Geometry: final body of the model. Coordinates: model frame, mm. A direction names the side the tool comes from. Give positions to 0.01 mm unless a question says otherwise; leave off trailing zeros. Order: outer loops, then holes, each group sorted by start corner. A loop starts at its lowest first (then second) coordinate and runs counter-clockwise, first axis right, second up. Notation, with made-up numbers: (-11, 5.25) -> (28, 5.25) arc R20 ccw to (28, 29.25) -> close; hole circle Ø2 at (-14.5, 77.5). An arc over 180 degrees is marked (long way). Answer in a Markdown table with one row per item. Add a question column.
Q1. Cut plane C-C on y = 2.25. Count the separate pieces of the cut face and the enclosed holes in it, and give its area (3 significant figures).
Q2. Set-up query: faces 4 (the face through (45, -4, 0)), 5 (the face through (-3.75, 2, -8)), 6 (the face through (19, 2.5, 10.5)). Return all of +Z, -Z, +X, -X, +Y, -Y with unobstructed straight access to the full face (end or side cutting, diameter ignored); none if empty.
Q3. Cut plane B-B on z = 0. Return the cut outline in (x, y), and give its area (3 significant figures).
Q4. Line query: line 1 along X through (y, z) = (1.6, 0); line 2 along X through (y, z) = (1.5, -8); line 3 along Z through (x, y) = (11.25, 1.25). Output: solid intervals per line, ascending. Write a range as from..to.
Q5. Contact query for flat-ended pins moving along their axis: P1, Ø1.5, axis at x = 10, y = 1.5, coming from the -Z side; P2, Ø2.5, axis at x = -10, y = 3.5, coming from the +Z side; P3, Ø1, axis at y = -2.5, z = -4, coming from the -X side; P4, Ø2, axis at x = 11.25, z = 0, coming from the -Y side. Output: stop coordinate, or through.
Q6. Cut plane D-D on x = 45.5. Return the cut outline in (y, z).
Q7. Pull-direction query (X, two-part tool) for faces 1 (the face through (11, 2, -9)), 2 (the face through (56.64, 2.54, 11.1)), 3 (the face through (-48.14, 2.54, 11.1)); classes: +X half, -X half, draft (parallel to the pull), parting line (faces both ways), or undercut.
Q8. Cut plane A-A on x = 11.25. Return the cut outline in (y, z).
from build123d import *

# Parameters (mm, degrees)
BOSS_EXTRUDE1_DEPTH = 5
SKETCH5_R           = 5
BOSS_EXTRUDE2_DEPTH = 4
SKETCH7_W           = 35
SKETCH7_H           = 3
CUT_EXTRUDE2_DEPTH  = 59.951251047
SKETCH6_W           = 7.5
SKETCH6_H           = 3
CUT_EXTRUDE1_DEPTH  = 59.951251047
SKETCH8_R           = 1.75
CUT_EXTRUDE3_DEPTH  = 59.951251047
FILLET3_R           = 3
FILLET2_R           = 0.25
CHAMFER1_SIZE       = 3


with BuildPart() as part:
    # Sketch1 → Boss-Extrude1 (new body)
    with BuildSketch(Plane(origin=(0, 0, 0), x_dir=(1, 0, 0), z_dir=(0, 1, 0))):
        Polygon((0, 12), (57.5, 12), (57.5, -12), (0, -12), (-49, -12), (-49, 12), align=None)
    extrude(amount=BOSS_EXTRUDE1_DEPTH)

    # Sketch5 → Boss-Extrude2 (add)
    with BuildSketch(Plane(origin=(0, 0, 0), x_dir=(1, 0, 0), z_dir=(0, 1, 0))):
        with Locations(Location((-37, 0, 0), (0, 0, 270))):
            Circle(SKETCH5_R)
        with Locations(Location((45.5, 0, 0), (0, 0, 90))):
            Circle(SKETCH5_R)
    extrude(amount=-BOSS_EXTRUDE2_DEPTH)

    # Sketch7 → Cut-Extrude2 (cut, through all)
    with BuildSketch(Plane.XZ):
        with Locations((0, 10.5)):
            Rectangle(SKETCH7_W, SKETCH7_H)
        with Locations((0, -10.5)):
            Rectangle(SKETCH7_W, SKETCH7_H)
    extrude(amount=-CUT_EXTRUDE2_DEPTH, mode=Mode.SUBTRACT)

    # Sketch6 → Cut-Extrude1 (cut, through all)
    with BuildSketch(Plane.XZ):
        with Locations((0, 7.5)):
            Rectangle(SKETCH6_W, SKETCH6_H)
        with Locations((0, -7.5)):
            Rectangle(SKETCH6_W, SKETCH6_H)
    extrude(amount=-CUT_EXTRUDE1_DEPTH, mode=Mode.SUBTRACT)

    # Sketch8 → Cut-Extrude3 (cut, through all)
    with BuildSketch(Plane.XZ):
        with Locations(Location((-11.25, 0, 0), (0, 0, 270))):
            Circle(SKETCH8_R)
        with Locations(Location((11.25, 0, 0), (0, 0, 90))):
            Circle(SKETCH8_R)
    extrude(amount=-CUT_EXTRUDE3_DEPTH, mode=Mode.SUBTRACT)

    # Fillet3
    fillet3_edges = [part.edges().sort_by_distance(p)[0] for p in [
        (-49, 2.5, 12),
        (-49, 2.5, -12),
        (57.5, 2.5, -12),
        (57.5, 2.5, 12),
    ]]
    fillet(fillet3_edges, radius=FILLET3_R)

    # Fillet2
    fillet2_edges = [part.edges().sort_by_distance(p)[0] for p in [
        (-37, -4, -5),
        (45.5, -4, 5),
    ]]
    fillet(fillet2_edges, radius=FILLET2_R)

    # Chamfer1
    chamfer1_edges = [part.edges().sort_by_distance(p)[0] for p in [
        (17.5, 2.5, 12),
        (-17.5, 2.5, 12),
        (17.5, 2.5, -12),
        (-17.5, 2.5, -12),
    ]]
    chamfer(chamfer1_edges, length=CHAMFER1_SIZE - 0.0001)  # a hair under: the kernel refuses the full size


solid = part.part
Completed:
| question | item | result |
|---|---|---|
| 1 | separate pieces | 1 |
| 1 | enclosed holes | 2 |
| 1 | area | 2,260 mm² |
| 2 | face 4 | +Z, -Z, +X, -X, -Y |
| 2 | face 5 | -Z, +Y, -Y |
| 2 | face 6 | +Z, +Y, -Y |
| 3 | outline | (-49, 0) -> (-42, 0) -> (-42, -3.75) arc R0.25 ccw to (-41.75, -4) -> (-32.25, -4) arc R0.25 ccw to (-32, -3.75) -> (-32, 0) -> (-13, 0) -> (-13, 5) -> (-49, 5) -> close; (-9.5, 0) -> (9.5, 0) -> (9.5, 5) -> (-9.5, 5) -> close; (13, 0) -> (40.5, 0) -> (40.5, -3.75) arc R0.25 ccw to (40.75, -4) -> (50.25, -4) arc R0.25 ccw to (50.5, -3.75) -> (50.5, 0) -> (57.5, 0) -> (57.5, 5) -> (13, 5) -> close |
| 3 | area | 577 mm² |
| 4 | line 1 | x = -49..-13, -9.5..9.5, 13..57.5 |
| 4 | line 2 | x = -49..-3.75, 3.75..57.5 |
| 4 | line 3 | z = -9..-1.75, 1.75..9 |
| 5 | P1 | stops at z = -9 |
| 5 | P2 | stops at z = 9 |
| 5 | P3 | stops at x = -40.57 |
| 5 | P4 | passes through |
| 6 | outline | (-4, -4.75) arc R0.25 ccw to (-3.75, -5) -> (0, -5) -> (0, -12) -> (5, -12) -> (5, 12) -> (0, 12) -> (0, 5) -> (-3.75, 5) arc R0.25 ccw to (-4, 4.75) -> close |
| 7 | face 1 | undercut |
| 7 | face 2 | +X half |
| 7 | face 3 | -X half |
| 8 | outline | (0, -9) -> (5, -9) -> (5, -1.75) -> (0, -1.75) -> close; (0, 1.75) -> (5, 1.75) -> (5, 9) -> (0, 9) -> close |
